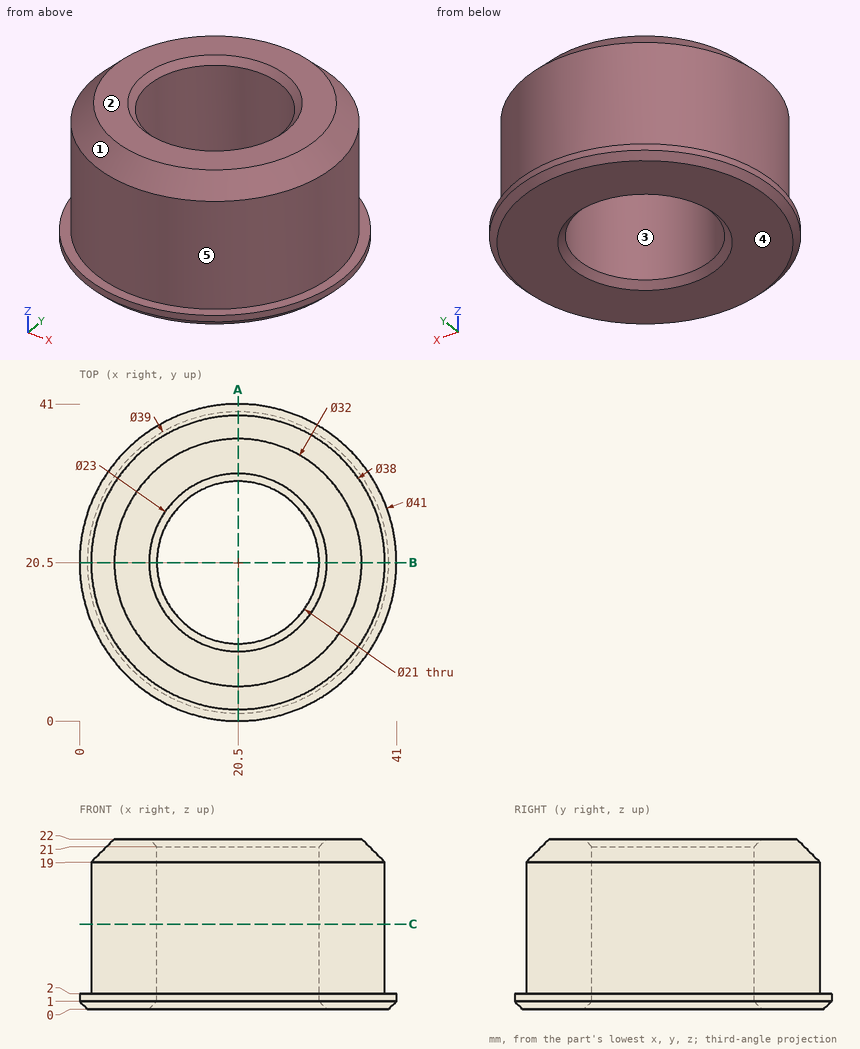
Input: dimensioned drawing with shaded views. Units: mm. Origin: part minimum x, y, z. A direction names the side the tool comes from. Give positions to 0.01 mm unless a question says otherwise; leave off trailing zeros. Write each loop counter-clockwise with the first axis right and the second up, starting at its lowest first coordinate (ties: lowest second). Pieces come first, ordered by that corner, then holes. Notation, with made-up numbers: (13.5, 35) -> (58.5, 35) arc R26 cw to (58.5, 49) -> close; hole circle Ø10 at (-33.75, 0). An arc over 180 degrees is marked (long way). Answer as a JSON object with one key per item and string values.
1. Contact query for flat-ended pins moving along their axis: pin 1 (12 mm diameter, centred on x = 19.5, z = 10, fed in from +Y); pin 2 (5 mm diameter, centred on y = 35.5, z = 18.5, fed in from -X); pin 3 (3 mm diameter, centred on x = 22, z = 2.5, fed in from +Y); pin 4 (6 mm diameter, centred on x = 15, y = 25, fed in from -Z). Output: stop coordinate, or through.
Ans:
{"pin 1": "stops at y = 39.5", "pin 2": "stops at x = 6.19", "pin 3": "stops at y = 41", "pin 4": "passes through"}
2. Access query for the marked faces 4 and 5. Directions: +Z, -Z, +X, -X, +Y, -Y. A direction counts if a zero-diameter tool reaches every point of the face in a straight line with its end or side. Return the directions, or none.
Ans:
{"face 4": "-Z, +X, -X, +Y, -Y", "face 5": "+Z"}
3. Cut plane A-A on x = 20.5. Output: boundary loops of the cut face in (y, z).
Ans:
{"outline": "(0, 1) -> (1, 0) -> (9, 0) -> (10, 1) -> (10, 21) -> (9, 22) -> (4.5, 22) -> (1.5, 19) -> (1.5, 2) -> (0, 2) -> close; (31, 1) -> (32, 0) -> (40, 0) -> (41, 1) -> (41, 2) -> (39.5, 2) -> (39.5, 19) -> (36.5, 22) -> (32, 22) -> (31, 21) -> close"}
4. Mould query, pull axis X, two halves, no side actions, for the marked faces 1, 2 and 3. Classes: pulls with the +X half, pulls with the -X half, needs draft (parallel to the pull), parting line crosses it, or undercut.
Ans:
{"face 1": "parting line crosses it", "face 2": "needs draft", "face 3": "undercut"}
5. Ray query, probe 1 along Y at (x, z) = (20.5, 10.5); probe 2 along Y at (x, z) = (15.5, 10); probe 3 along X at (y, z) = (26, 16). Return the intervals inside material, ascending. Write a range as from..to.
Ans:
{"probe 1": "y = 1.5..10, 31..39.5", "probe 2": "y = 2.17..11.27, 29.73..38.83", "probe 3": "x = 2.31..11.56, 29.44..38.69"}
6. Cut plane C-C on z = 11. Output: boundary loops of the cut face in (x, y).
Ans:
{"outline": "circle Ø38 at (20.5, 20.5); hole circle Ø21 at (20.5, 20.5)"}
